The listing builds one solid part. Answer for the finished solid, in the listing's coordinates (mm). Face numbers are marked on the shaded views. A direction names the side the tool comes from. Give positions to 0.01 mm unless a question says otherwise; leave off trailing zeros. Answer as CSV lines item,"result". Start each with the question number.
1) For the marked faces 1, 2 and 3, determine the directions among +Z, -Z, +X, -X, +Y, -Y from which every point of the face is accessible in a straight line to the end or side of a thin tool.
2) Find the intervals of material crossed by line 1 along Y through (x, z) = (26, -28); line 2 along Y through (x, z) = (0, -33); line 3 along X through (y, z) = (0.5, -26), in increasing order.
3) A cutting plane is placed at B-B (y = 0). Give the number of separate pieces and of enclosed holes in the cut face, and give its area (3 significant figures).
4) Flat-ended cylindrical pins translate along their axes: pin 1 (3 mm diameter, centred on x = 23.5, z = 8.5, fed in from -Y); pin 2 (4 mm diameter, centred on y = -22.5, z = -25, fed in from -X); pin 3 (14.5 mm diameter, centred on x = 0, y = 6, fed in from -Z) (3 decimals); pin 4 (20 mm diameter, centred on x = 0, y = 0, fed in from +Z). Find the tip coordinate at first contact, or state that the pin passes through.
5) For a pull along X with two mould halves and no side action, classify the marked faces 4, 5 and 6 as pulls with the +X half, pulls with the -X half, needs draft (parallel to the pull), parting line crosses it, or undercut.
Autodesk Inventor part; units mm, degrees
ref_plane "YZ Plane" through (0, 0, 0) normal (1, 0, 0) x (0, 1, 0)
ref_plane "XZ Plane" through (0, 0, 0) normal (0, 1, 0) x (-1, 0, 0)
ref_plane "XY Plane" through (0, 0, 0) normal (0, 0, 1) x (1, 0, 0)
sketch "Sketch1" plane through (0, 0, 0) normal (0, 0, 1) x (1, 0, 0)
  circle A0 centre (0, 0) radius 11.1125
  circle A1 centre (0, 0) radius 57.15 construction
  line L0 (29.571, 44.45) -> (35.921, 44.45) construction
  line L1 (35.921, 44.45) -> (35.921, -44.45) construction
  line L2 (35.921, -44.45) -> (29.571, -44.45) construction
  line L3 (29.571, -44.45) -> (29.571, 44.45) construction
  line L4 (31.75, 47.519) -> (31.75, -47.519)
  arc A2 (31.75, 47.519) -> (31.75, -47.519) centre (0, 0) ccw
  point P0 (29.571, 0)
  point P1 (57.15, 0)
  point P2 (35.921, 0)
  dimension "d0" = 22.225
  dimension "d2" = 114.3
  dimension "d3" = 88.9
  dimension "d4" = 6.35
  dimension "d5" = 35.921
  dimension "d6" = 21.229
  dimension "d7" = 31.75
extrude "Extrusion1" add sketch "Sketch1" along normal mid plane 82.55
sketch "Sketch3" plane through (0, 0, 41.275) normal (0, 0, 1) x (1, 0, 0)
  circle A0 centre (0, 0) radius 11.1125 construction
  arc A1 (31.75, 47.519) -> (31.75, -47.519) centre (0, 0) ccw construction
  line L0 (31.75, 47.519) -> (31.75, -47.519) construction
  circle A2 centre (0, 0) radius 11.1125 construction
  circle A3 centre (0, 0) radius 23.8125
  dimension "d10" = 47.625
extrude "Extrusion2" cut sketch "Sketch3" against normal blind 12.7
sketch "Sketch4" plane through (0, 0, -41.275) normal (0, 0, -1) x (-1, 0, 0)
  circle A0 centre (0, 0) radius 23.8125
  dimension "d13" = 47.625
extrude "Extrusion3" cut sketch "Sketch4" against normal blind 12.7
sketch "Sketch5" plane through (31.75, -47.519, 41.275) normal (1, 0, 0) x (0, 0, -1)
  line L0 (82.55, 95.0381) -> (82.55, 0) construction
  line L1 (82.55, 0) -> (0, 0) construction
  line L2 (0, 0) -> (0, 95.0381) construction
  line L3 (0, 95.0381) -> (82.55, 95.0381) construction
  circle A0 centre (41.275, 47.519) radius 38.1 construction
  point P0 (41.275, 85.619)
  point P1 (14.3342, 74.4598)
  point P2 (3.175, 47.519)
  point P3 (14.3342, 20.5783)
  point P4 (41.275, 9.419)
  point P5 (68.2158, 20.5783)
  point P6 (79.375, 47.519)
  point P7 (68.2158, 74.4598)
  dimension "d16" = 76.2
  dimension "d32" = 360
hole "Hole1" at (31.75, 26.9408, -26.9408) at (31.75, 0, -38.1) at (31.75, 26.9408, 26.9408) at (31.75, 0, 38.1) at (31.75, -26.9408, 26.9408) at (31.75, -26.9408, -26.9408) direction (-1, 0, 0) diameter 3.9624 depth 13.6144
pattern_circular "Circular Pattern1" [suppressed]
sketch "Sketch6" plane through (0, 0, 41.275) normal (0, 0, 1) x (1, 0, 0)
  circle A0 centre (0, 0) radius 23.8125 construction
  arc A1 (31.75, 47.519) -> (31.75, -47.519) centre (0, 0) ccw construction
  line L0 (31.75, 47.519) -> (31.75, -47.519) construction
  circle A2 centre (0, 0) radius 44.45
  circle A3 centre (0, 0) radius 57.15
  arc A4 (31.75, 47.519) -> (31.75, -47.519) centre (0, 0) ccw construction
  dimension "d27" = 12.7
extrude "Extrusion4" cut sketch "Sketch6" against normal through all
equation "\"d13\" = d10"
equation "\"d14\" = d11"
properties part number "EL2-A-004" material "Aluminum 6061"
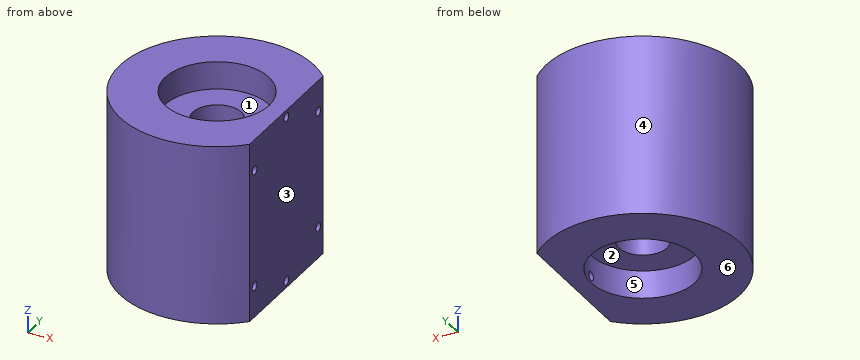
Ans:
1,face 1,"+Z"
1,face 2,"-Z"
1,face 3,"+Z, -Z, +X, +Y, -Y"
2,line 1,"-36.05 to -28.62, -25.27 to 25.27, 28.62 to 36.05"
2,line 2,"-44.45 to -23.81, 23.81 to 44.45"
2,line 3,"-44.45 to -11.1, 11.1 to 31.75"
3,separate pieces,"4"
3,enclosed holes,"0"
3,area,"3,750 mm2"
4,pin 1,"y = -38.62"
4,pin 2,"x = -39.44"
4,pin 3,"z = -28.575"
4,pin 4,"through"
5,face 4,"parting line crosses it"
5,face 5,"undercut"
5,face 6,"needs draft"
